```python
from build123d import *

# Parameters (mm, degrees)
SKETCH1_R               = 25.4
BOSS_EXTRUDE1_DEPTH     = 2.54
SKETCH2_R               = 6.35
BOSS_EXTRUDE2_DEPTH     = 152.4
SKETCH3_R               = 9.525
BOSS_EXTRUDE3_DEPTH     = 22.86
CUT_EXTRUDE2_DEPTH      = 160.049437597
CUT_EXTRUDE2_DEPTH_BACK = 160.049437597
SKETCH4_W               = 3.175
SKETCH4_H               = 19.05
CUT_EXTRUDE3_DEPTH      = 161.18622319
CUT_EXTRUDE3_DEPTH_BACK = 161.18622319
SKETCH5_R               = 4.7625


with BuildPart() as part:
    # Sketch1 → Boss-Extrude1 (new body)
    with BuildSketch(Plane.XY):
        Circle(SKETCH1_R)
    extrude(amount=BOSS_EXTRUDE1_DEPTH)

    # Sketch2 → Boss-Extrude2 (add)
    with BuildSketch(Plane.XY.offset(2.54)):
        with Locations(Location((0, 0, 0), (0, 0, 180))):
            Circle(SKETCH2_R)
    extrude(amount=BOSS_EXTRUDE2_DEPTH)

    # Sketch3 → Boss-Extrude3 (add)
    with BuildSketch(Plane(origin=(0, 0, 0), x_dir=(-1, 0, 0), z_dir=(0, 0, -1))):
        Circle(SKETCH3_R)
    extrude(amount=BOSS_EXTRUDE3_DEPTH)

    # Sketch4 → Cut-Extrude2 (cut, two sides: drawn at the far end of the back side and taken through both)
    with BuildSketch(Plane(origin=(0, 0, 0), x_dir=(1, 0, 0), z_dir=(0, 1, 0)).offset(-CUT_EXTRUDE2_DEPTH_BACK)):
        with Locations((7.9375, 13.335)):
            Rectangle(SKETCH4_W, SKETCH4_H)
        with Locations((-7.9375, 13.335)):
            Rectangle(SKETCH4_W, SKETCH4_H)
    extrude(amount=CUT_EXTRUDE2_DEPTH + CUT_EXTRUDE2_DEPTH_BACK, mode=Mode.SUBTRACT)

    # Sketch5 → Cut-Extrude3 (cut, two sides: drawn at the far end of the back side and taken through both)
    with BuildSketch(Plane.ZY.offset(6.35).offset(-CUT_EXTRUDE3_DEPTH_BACK)):
        with Locations((-13.335, 0)):
            Circle(SKETCH5_R)
    extrude(amount=CUT_EXTRUDE3_DEPTH + CUT_EXTRUDE3_DEPTH_BACK, mode=Mode.SUBTRACT)


solid = part.part
```
Geometry: final body of the model. Coordinates: model frame, mm. A direction names the side the tool comes from. Coordinates: 2 decimals unless noted, no trailing zeros. Loops run counter-clockwise (first coordinate to the right, second up) from the corner with the lowest first, then second, coordinate; pieces in that order, holes last. Notation, with made-up numbers: M 25.25,9.5 L 39.25,9.5 A25 cw 39.25,21.5 Z; hole C 64.25,35 d11. An arc over 180 degrees is marked long. Put each result on its own line as item: value.
(1) First-contact query: pin 1 (6 mm diameter, centred on y = -4.5, z = 74.5, fed in from -X); pin 2 (7 mm diameter, centred on y = 0, z = -14, fed in from +X); pin 3 (8 mm diameter, centred on x = -19.5, y = -12, fed in from -Z); pin 4 (12 mm diameter, centred on y = 4, z = 128, fed in from -X). Flat tips, straight axial feed; report the tip coordinate or a pass-through.
Answer sheet:
pin 1: stops at x = -6.17
pin 2: passes through
pin 3: stops at z = 0
pin 4: stops at x = -6.35
(2) Draft query along Z for faces 1 (the face through (11, 0, 0)), 2 (the face through (0.089, 3.219, -16.845)), 3 (the face through (-6.35, -5, -13)). Return one class per face: pulls with the +Z half, pulls with the -Z half, needs draft (parallel to the pull), parting line crosses it, or undercut.
Answer sheet:
face 1: pulls with the -Z half
face 2: undercut
face 3: needs draft
(3) Material intervals for probe 1 along Z at (x, y) = (-0.25, 0); probe 2 along Z at (x, y) = (0.5, -9); probe 3 along Z at (x, y) = (-22.5, -10.5), sorted ascending.
Answer sheet:
probe 1: z = -22.86 to -18.1, -8.57 to 154.94
probe 2: z = -22.86 to 2.54
probe 3: z = 0 to 2.54
(4) Access query for faces 4 (the face through (6.35, -5, -13)), 5 (the face through (-8, 0, -3.81)), 6 (the face through (0, 0, 154.94)), 7 (the face through (-2.93, 5.634, 77.673)), 8 (the face through (-5.12, 8.03, -8.73)). Directions: +Z, -Z, +X, -X, +Y, -Y. A direction counts if a zero-diameter tool reaches every point of the face in a straight line with its end or side. Return the directions, or none.
Answer sheet:
face 4: -Z, +X, +Y, -Y
face 5: -Z, -X, +Y, -Y
face 6: +Z, +X, -X, +Y, -Y
face 7: +Z
face 8: -Z
(5) Cut plane D-D on y = -14.5. Return the cut outline in (x, z), then the cut area to 3 significant figures.
Answer sheet:
outline: M -20.85,0 L 20.85,0 L 20.85,2.54 L -20.85,2.54 Z
area: 106 mm^2
(6) Cut plane C-C on z = 142. Return the cut outline in (x, y), then the cut area to 3 significant figures.
Answer sheet:
outline: C 0,0 d12.7
area: 127 mm^2
